The model under review builds one solid part; all positions refer to its coordinate system, in mm. Face numbers are marked on the shaded views. A direction names the side the tool comes from. Coordinates: 2 decimals unless noted, no trailing zeros. Write each loop counter-clockwise with the first axis right and the second up, starting at its lowest first coordinate (ties: lowest second). Pieces come first, ordered by that corner, then holes. Notation, with made-up numbers: M 62.5,83 L 88.5,83 A31 ccw 88.5,122 Z; hole C -4.75,26 d8. An arc over 180 degrees is marked long. Answer as a JSON object with one key per item and string values.
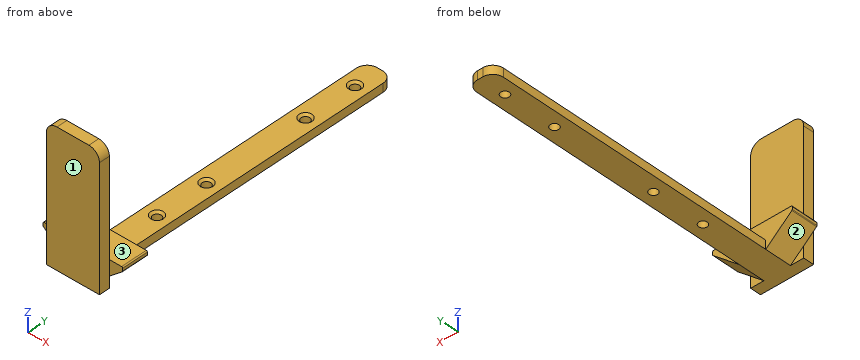
```python
from build123d import *

# Parameters (mm, degrees)
F0_W     = 6.35
F0_H     = 76.2
F0_R     = 1.016
F1_DEPTH = 2.032
F3_DEPTH = 6.35
F4_R     = 0.254
F5_R     = 0.254
F6_SIZE  = 0.508
F7_SIZE  = 0.508
F8_W     = 12.7
F8_H     = 25.4
F9_DEPTH = 2.54
F10_R    = 2.54
F11_R    = 2.54


with BuildPart() as f1:
    # F0 (on Top) → F1 (new body)
    with BuildSketch(Plane.XY):
        with Locations((0, 28.9922469051)):
            Rectangle(F0_W, F0_H)
        with Locations((0, 9.9422469051)):
            Circle(F0_R, mode=Mode.SUBTRACT)
        with Locations((0, 22.6422469051)):
            Circle(F0_R, mode=Mode.SUBTRACT)
        with Locations((0, 48.0422469051)):
            Circle(F0_R, mode=Mode.SUBTRACT)
        with Locations((0, 60.7422469051)):
            Circle(F0_R, mode=Mode.SUBTRACT)
    extrude(amount=F1_DEPTH)

    # F2 (on face) → F3 (join)
    with BuildSketch(Plane.XZ.offset(9.1077530949)):
        Polygon((-9.525, 5.3878031066), (-3.175, 0), (3.175, 0), (9.525, 5.3573960435), (9.525, 6.35), (3.175, 6.35), (-3.175, 6.35), (-9.525, 6.35), align=None)
    extrude(amount=-F3_DEPTH)

    # F4
    f4_edges = [f1.edges().sort_by_distance(p)[0] for p in [
        (9.525, -5.932753, 6.35),
    ]]
    fillet(f4_edges, radius=F4_R)

    # F5
    f5_edges = [f1.edges().sort_by_distance(p)[0] for p in [
        (9.525, -5.932753, 5.357396),
        (-9.525, -5.932753, 6.35),
        (-9.525, -5.932753, 5.387803),
    ]]
    fillet(f5_edges, radius=F5_R)

    # F6
    f6_edges = [f1.edges().sort_by_distance(p)[0] for p in [
        (-1.016, 60.742247, 2.032),
    ]]
    chamfer(f6_edges, length=F6_SIZE)

    # F7
    f7_edges = [f1.edges().sort_by_distance(p)[0] for p in [
        (-1.016, 48.042247, 2.032),
        (-1.016, 22.642247, 2.032),
        (-1.016, 9.942247, 2.032),
    ]]
    chamfer(f7_edges, length=F7_SIZE)

    # F8 (on face) → F9 (join)
    with BuildSketch(Plane.XZ.offset(9.1077530949)):
        with Locations((0, 19.05)):
            Rectangle(F8_W, F8_H)
        Polygon((6.35, 6.35), (-6.35, 6.35), (-6.35, 2.6939015533), (-3.175, 0), (3.175, 0), (6.35, 2.6786980217), align=None)
        Polygon((6.35, 0), (6.35, 2.6786980217), (3.175, 0), align=None)
        Polygon((-3.175, 0), (-6.35, 2.6939015533), (-6.35, 0), align=None)
    extrude(amount=F9_DEPTH)

    # F10
    f10_edges = [f1.edges().sort_by_distance(p)[0] for p in [
        (6.35, -10.377753, 31.75),
        (-6.35, -10.377753, 31.75),
    ]]
    fillet(f10_edges, radius=F10_R)

    # F11
    f11_edges = [f1.edges().sort_by_distance(p)[0] for p in [
        (-3.175, 67.092247, 1.016),
        (3.175, 67.092247, 1.016),
    ]]
    fillet(f11_edges, radius=F11_R)


solid = f1.part
```
(1) For the marked faces 1, 2 and 3, list the 3-axis set-ups (+Z, -Z, +X, -X, +Y, -Y) from which the entire face can be reached by the end or side of a thin tool; tool diameter is ignored.
Results list:
{"face 1": "+Z, -Z, +X, -X, -Y", "face 2": "-Z, -X, +Y", "face 3": "+Z, +X, -X, +Y"}
(2) Wall thickness on line 1 along Y through (x, z) = (0, 1.25); line 2 along Z through (x, y) = (1, -8); line 3 along Z through (x, y) = (1, 38): over which ranges is each line inside the solid? List them lowest first. Write a range as from..to.
Results list:
{"line 1": "-11.65..8.93, 10.96..21.63, 23.66..47.03, 49.06..59.73, 61.76..67.09", "line 2": "0..6.35", "line 3": "0..2.03"}
(3) Add section B-B on z = 13. Give the boundary of the cut face in (x, y), and give its area (3 significant figures).
Results list:
{"outline": "M -6.35,-11.65 L 6.35,-11.65 L 6.35,-9.11 L -6.35,-9.11 Z", "area": "32.3 mm²"}
(4) For pin 1 Ø4 at (y, z) = (7.5, 4.5) entering from +X; pin 2 Ø2.5 at (x, y) = (0, 22.64) entering from +Z; pin 3 Ø10 at (x, y) = (-4.5, 51) entering from +Z; pin 4 Ø3 at (x, y) = (3.5, -1.5) entering from +Z, all flat-tipped, find the tip position at first contact; note any pin that passes through.
Results list:
{"pin 1": "through", "pin 2": "z = 1.76", "pin 3": "z = 2.03", "pin 4": "z = 6.35"}
(5) Add section A-A on y = 30.5. Give the boundary of the cut face in (x, z) (3 decimals), and give its area (3 significant figures).
Results list:
{"outline": "M -3.175,0 L 3.175,0 L 3.175,2.032 L -3.175,2.032 Z", "area": "12.9 mm²"}
